```python
from build123d import *

# Parameters (mm, degrees)
SKETCH_1_W           = 210
SKETCH_1_H           = 233
EXTRUDE_1_DEPTH      = 1
SKETCH_2_R           = 65
CUT_EXTRUDE_1_DEPTH  = 2
SKETCH_3_W           = 210
SKETCH_3_H           = 16.25
CUT_EXTRUDE_2_DEPTH  = 2
SKETCH_4_W           = 210
SKETCH_4_H           = 0.1
CUT_EXTRUDE_3_DEPTH  = 2
CUT_EXTRUDE_4_DEPTH  = 2
SKETCH_8_R           = 1.6
CUT_EXTRUDE_6_DEPTH  = 1
SKETCH_12_R          = 1.35
CUT_EXTRUDE_9_DEPTH  = 10
CUT_EXTRUDE_10_DEPTH = 10
FILLET_3_R           = 2
SKETCH_15_R          = 1.6
CUT_EXTRUDE_12_DEPTH = 10
SKETCH_17_R          = 1.55
CUT_EXTRUDE_13_DEPTH = 10
CUT_EXTRUDE_14_DEPTH = 10
FILLET_6_R           = 5
SKETCH_24_W          = 210
SKETCH_24_H          = 18.25
CUT_EXTRUDE_18_DEPTH = 10


with BuildPart() as part:
    # 草图1 → 凸台-拉伸1 (new body)
    with BuildSketch(Plane.XY):
        Rectangle(SKETCH_1_W, SKETCH_1_H)
    extrude(amount=EXTRUDE_1_DEPTH)

    # 草图2 → 切除-拉伸1 (cut)
    with BuildSketch(Plane.XY.offset(1)):
        with Locations((-15, 100.25)):
            Circle(SKETCH_2_R)
    extrude(amount=-CUT_EXTRUDE_1_DEPTH, mode=Mode.SUBTRACT)

    # 草图3 → 切除-拉伸2 (cut)
    with BuildSketch(Plane.XY.offset(1)):
        with Locations((0, 108.375)):
            Rectangle(SKETCH_3_W, SKETCH_3_H)
    extrude(amount=-CUT_EXTRUDE_2_DEPTH, mode=Mode.SUBTRACT)

    # 草图4 → 切除-拉伸3 (cut)
    with BuildSketch(Plane.XY.offset(1)):
        with Locations((0, 100.2)):
            Rectangle(SKETCH_4_W, SKETCH_4_H)
    extrude(amount=-CUT_EXTRUDE_3_DEPTH, mode=Mode.SUBTRACT)

    # 草图5 → 切除-拉伸4 (cut)
    with BuildSketch(Plane.XY.offset(1)):
        with BuildLine():
            Line((4.5, 38.243951908), (95.5, 66.86212795))
            ThreePointArc((95.5, 66.86212795), (105.715966735, 128.460790883), (50.000008252, 100.274034742))
            Line((50.000008252, 100.274034742), (49.999923077, 100.15))
            ThreePointArc((49.999923077, 100.15), (37.375079452, 61.755181486), (4.5, 38.243951908))
        make_face()
    extrude(amount=-CUT_EXTRUDE_4_DEPTH, mode=Mode.SUBTRACT)

    # 草图8 → 切除-拉伸6 (cut)
    with BuildSketch(Plane.XY.offset(1)):
        with Locations((-100, -21.5)):
            Circle(SKETCH_8_R)
        with Locations((-100, -1.5)):
            Circle(SKETCH_8_R)
    extrude(amount=-CUT_EXTRUDE_6_DEPTH, mode=Mode.SUBTRACT)

    # 草图12 → 切除-拉伸9 (cut)
    with BuildSketch(Plane(origin=(0, 0, 0), x_dir=(-1, 0, 0), z_dir=(0, 0, -1))):
        with Locations((-18.75, -13.7)):
            Circle(SKETCH_12_R)
        with Locations((48.75, -13.7)):
            Circle(SKETCH_12_R)
        with Locations((-7, -69.7)):
            Circle(SKETCH_12_R)
        with Locations((37, -69.7)):
            Circle(SKETCH_12_R)
    extrude(amount=-CUT_EXTRUDE_9_DEPTH, mode=Mode.SUBTRACT)

    # 草图13 → 切除-拉伸10 (cut)
    with BuildSketch(Plane(origin=(0, 0, 0), x_dir=(-1, 0, 0), z_dir=(0, 0, -1))):
        with BuildLine():
            Line((7.5, -84.7), (22.5, -84.7))
            ThreePointArc((22.5, -84.7), (27.5, -89.7), (22.5, -94.7))
            Line((22.5, -94.7), (7.5, -94.7))
            ThreePointArc((7.5, -94.7), (2.5, -89.7), (7.5, -84.7))
        make_face()
    extrude(amount=-CUT_EXTRUDE_10_DEPTH, mode=Mode.SUBTRACT)

    # 圆角3
    fillet_3_edges = [part.edges().sort_by_distance(p)[0] for p in [
        (105, 71.527186767, 0.5),
        (-79.999923077, 100.15, 0.5),
        (-105, 100.15, 0.5),
        (105, -116.5, 0.5),
        (-105, -116.5, 0.5),
    ]]
    fillet(fillet_3_edges, radius=FILLET_3_R)

    # 草图15 → 切除-拉伸12 (cut)
    with BuildSketch(Plane(origin=(0, 0, 0), x_dir=(-1, 0, 0), z_dir=(0, 0, -1))):
        with Locations((-32.5, -85.75)):
            Circle(SKETCH_15_R)
        with Locations((-32.5, -93.25)):
            Circle(SKETCH_15_R)
        with Locations((62.5, -85.75)):
            Circle(SKETCH_15_R)
        with Locations((62.5, -93.25)):
            Circle(SKETCH_15_R)
    extrude(amount=-CUT_EXTRUDE_12_DEPTH, mode=Mode.SUBTRACT)

    # 草图17 → 切除-拉伸13 (cut)
    with BuildSketch(Plane(origin=(0, 0, 0), x_dir=(-1, 0, 0), z_dir=(0, 0, -1))):
        with Locations((-101, -49.75)):
            Circle(SKETCH_17_R)
        with Locations((-101, -69.75)):
            Circle(SKETCH_17_R)
    extrude(amount=-CUT_EXTRUDE_13_DEPTH, mode=Mode.SUBTRACT)

    # 草图18 → 切除-拉伸14 (cut)
    with BuildSketch(Plane(origin=(0, 0, 0), x_dir=(-1, 0, 0), z_dir=(0, 0, -1))):
        with BuildLine():
            Line((-92.5, 50.815700167), (5.25, 35.985410217))
            Line((5.25, 35.985410217), (-105, 79.42424305))
            Line((-105, 79.42424305), (-105, 54.42424305))
            ThreePointArc((-105, 54.42424305), (-98.86787278, 52.211660056), (-92.5, 50.815700167))
        make_face()
    extrude(amount=-CUT_EXTRUDE_14_DEPTH, mode=Mode.SUBTRACT)

    # 圆角6
    fillet_6_edges = [part.edges().sort_by_distance(p)[0] for p in [
        (105, 54.42424305, 0.5),
    ]]
    fillet(fillet_6_edges, radius=FILLET_6_R)

    # 草图24 → 切除-拉伸18 (cut)
    with BuildSketch(Plane.XY.offset(1)):
        with Locations((0, -107.375)):
            Rectangle(SKETCH_24_W, SKETCH_24_H)
    extrude(amount=-CUT_EXTRUDE_18_DEPTH, mode=Mode.SUBTRACT)


solid = part.part
```
Verification items for the finished model (mm, model axes). A direction names the side the tool comes from. Give positions to 0.01 mm unless a question says otherwise; leave off trailing zeros. Loops run counter-clockwise (first coordinate to the right, second up) from the corner with the lowest first, then second, coordinate; pieces in that order, holes last.
1. Go/stop test with a flat-tipped pin: pin 1 Ø2.5 at (x, y) = (101, -49.75) entering from +Z. Record where the tip stops, or that it passes through.
2. Set-up check for faces 3 (the flat face through (-1, -20, 0)), 4 (the cylindrical face through (-2.5, -89.8, 0.5)), 5 (the flat face through (44.309, 43.504, 0.493)): record each of +Z, -Z, +X, -X, +Y, -Y from which the full face is reachable in a straight line by a thin tool's end or side.
3. Section check A-A, the plane z = 0.15. Count the separate pieces of the cut face and the enclosed holes in it, then the cut area to 3 significant figures.
4. Mould release check, pull along X, two halves, no side actions. Record for faces 1 (the flat face through (-1, -20, 1)), 2 (the cylindrical face through (-57.185, 50.799, 0.507)): released by +X, released by -X, zero draft, split by the parting line, or undercut.
5. Thickness scan on line 1 (Y direction, x = -100, z = 0.35); line 2 (X direction, y = -69.7, z = 0.7); line 3 (Y direction, x = 32.5, z = 0.55). Record the ranges inside material, lowest first.
6. Section check B-B, the plane y = 58.5. Enter the section's corners in (x, z).
Geometry says:
1. pin 1: passes through
2. face 3: -Z, +X, -X, +Y, -Y
2. face 4: +Z, -Z
2. face 5: +Z, -Z, +Y
3. separate pieces: 1
3. enclosed holes: 13
3. area: 31,200 mm2
4. face 1: zero draft
4. face 2: undercut
5. line 1: y = -98.25 to -23.1, -19.9 to -3.1, 0.1 to 100.15
5. line 2: x = -105 to -38.35, -35.65 to 5.65, 8.35 to 99.45, 102.55 to 105
5. line 3: y = -98.25 to -94.85, -91.65 to -87.35, -84.15 to 41.71
6. outline: (-105, 0) - (-64.82, 0) - (-64.82, 1) - (-105, 1) - close
